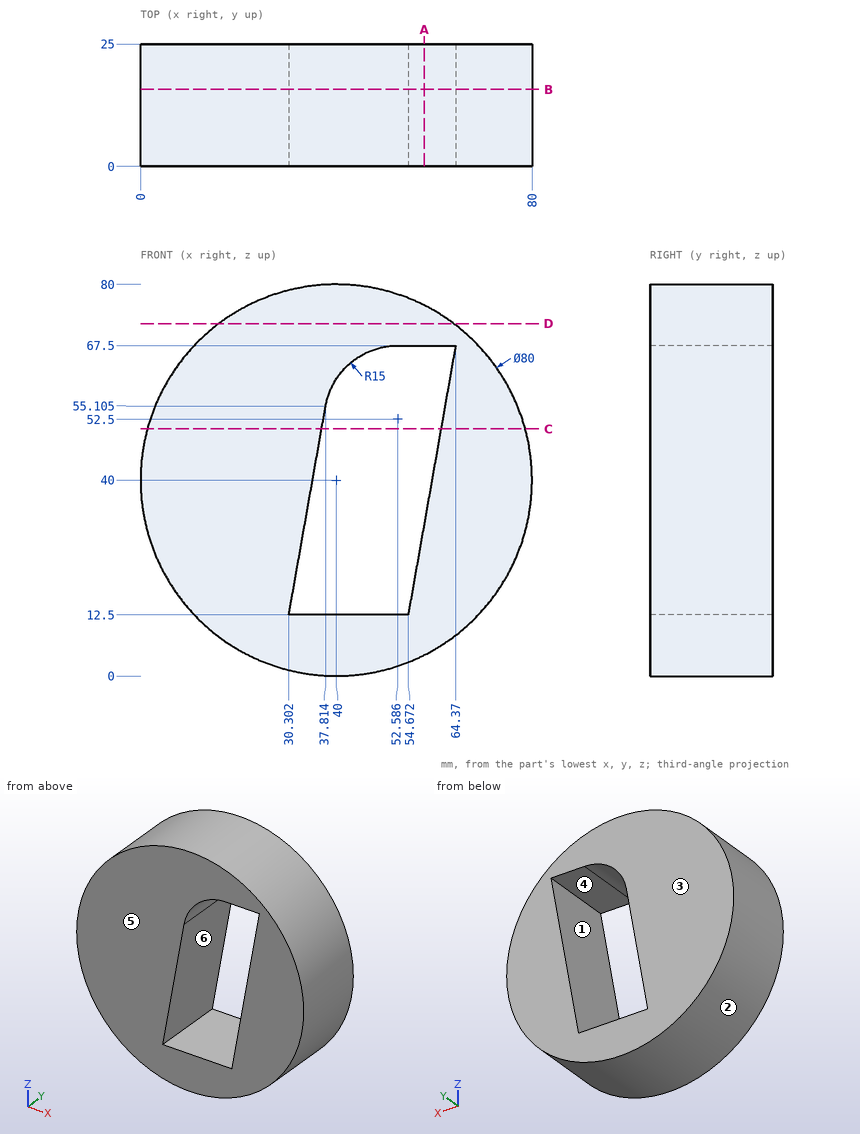
Design review of the part shown in the three views and the two pictorial views. Dimensions are in mm from the part's minimum x, y and z. A direction names the side the tool comes from. Round coordinates to 2 decimals unless told otherwise and drop trailing zeros. Loops run counter-clockwise (first coordinate to the right, second up) from the corner with the lowest first, then second, coordinate; pieces in that order, holes last. Notation, with made-up numbers: (71, 45) - (112, 45) arc R21 ccw to (112, 80) - close; hole circle Ø8 at (-15.75, 89). An arc over 180 degrees is marked (long way). Use one line per item in the form item = value.
1) We need section C-C on z = 50.5. Write out the cut boundary in (x, y), then the cut area to 3 significant figures.
Solutions:
outline = (1.4, 0) - (37, 0) - (37, 25) - (1.4, 25) - close; (61.37, 0) - (78.6, 0) - (78.6, 25) - (61.37, 25) - close
area = 1,320 mm2
2) Tool access review of the marked faces 5 and 6: name each direction out of +Z, -Z, +X, -X, +Y, -Y from which nothing blocks a thin tool from reaching the whole face with its end or side.
Solutions:
face_5 = +Z, -Z, +X, -X, -Y
face_6 = +Y, -Y
3) We need section A-A on x = 58. Write out the cut boundary in (y, z).
Solutions:
outline = (0, 4.28) - (25, 4.28) - (25, 31.37) - (0, 31.37) - close; (0, 67.5) - (25, 67.5) - (25, 75.72) - (0, 75.72) - close
4) Clearance check with flat-ended pins moving along their axes: P1, Ø5, axis at x = 23, y = 9.5, coming from the +Z side; P2, Ø3.5, axis at x = 60.5, y = 15.5, coming from the -Z side; P3, Ø7.5, axis at x = 38.5, y = 18, coming from the +Z side. State where each tip first meets the part, or that it passes through.
Solutions:
P1 = 77.28
P2 = 4.67
P3 = 80
5) We need section D-D on z = 72. Write out the cut boundary in (x, y), then the cut area to 3 significant figures.
Solutions:
outline = (16, 0) - (64, 0) - (64, 25) - (16, 25) - close
area = 1,200 mm2
6) We need section B-B on y = 15.75. Write out the cut boundary in (x, z) (1 decimal).
Solutions:
outline = circle Ø80 at (40, 40); hole (30.3, 12.5) - (54.7, 12.5) - (64.4, 67.5) - (52.6, 67.5) arc R15 ccw to (37.8, 55.1) - close
7) Mouldability with a two-part tool opening along X and no side actions: class the marked faces 1, 2, 3 and 4 as pulls with the +X half, pulls with the -X half, needs draft (parallel to the pull), parting line crosses it, or undercut.
Solutions:
face_1 = undercut
face_2 = parting line crosses it
face_3 = needs draft
face_4 = undercut
8) Wall thickness on probe 1 along X at (y, z) = (17.75, 15.5); probe 2 along X at (y, z) = (23.25, 27.5); probe 3 along Z at (x, y) = (39, 11.5) (1 decimal): over which ranges is each line inside the solid? List them lowest first.
Solutions:
probe_1 = 8.38 to 30.83, 55.2 to 71.62
probe_2 = 2 to 32.95, 57.32 to 78
probe_3 = 0 to 12.5, 58.9 to 80
